from build123d import *

# Parameters (mm, degrees)
BOSS_EXTRUDE1_DEPTH = 3
FILLET1_R           = 10
FILLET2_R           = 1
FILLET3_R           = 3
SKETCH2_R           = 2.1
CUT_EXTRUDE1_DEPTH  = 42.12177039


with BuildPart() as part:
    # Sketch1 → Boss-Extrude1 (new body)
    with BuildSketch(Plane(origin=(0, 0, 0), x_dir=(1, 0, 0), z_dir=(0, 1, 0))):
        Polygon((29, -17.5), (25, -17.5), (25, -29), (-25, -29), (-25, -17.5), (-29, -17.5), (-29, 17.5), (-25, 17.5), (-25, 29), (25, 29), (25, 17.5), (29, 17.5), align=None)
    extrude(amount=BOSS_EXTRUDE1_DEPTH)

    # Fillet1
    fillet1_edges = [part.edges().sort_by_distance(p)[0] for p in [
        (25, 1.5, 29),
        (-25, 1.5, 29),
        (-25, 1.5, -29),
        (25, 1.5, -29),
    ]]
    fillet(fillet1_edges, radius=FILLET1_R)

    # Fillet2
    fillet2_edges = [part.edges().sort_by_distance(p)[0] for p in [
        (25, 1.5, 17.5),
        (-25, 1.5, 17.5),
        (-25, 1.5, -17.5),
        (25, 1.5, -17.5),
    ]]
    fillet(fillet2_edges, radius=FILLET2_R)

    # Fillet3
    fillet3_edges = [part.edges().sort_by_distance(p)[0] for p in [
        (29, 1.5, 17.5),
        (29, 1.5, -17.5),
        (-29, 1.5, 17.5),
        (-29, 1.5, -17.5),
    ]]
    fillet(fillet3_edges, radius=FILLET3_R - 0.0001)  # a hair under: the kernel refuses the full size

    # Sketch2 → Cut-Extrude1 (cut, through all)
    with BuildSketch(Plane(origin=(0, 3, 0), x_dir=(1, 0, 0), z_dir=(0, 1, 0))):
        with Locations(Location((-25.2, 0, 0), (0, 0, 270))):
            Circle(SKETCH2_R)
        with Locations(Location((25.2, 0, 0), (0, 0, 270))):
            Circle(SKETCH2_R)
    extrude(amount=-CUT_EXTRUDE1_DEPTH, mode=Mode.SUBTRACT)


solid = part.part
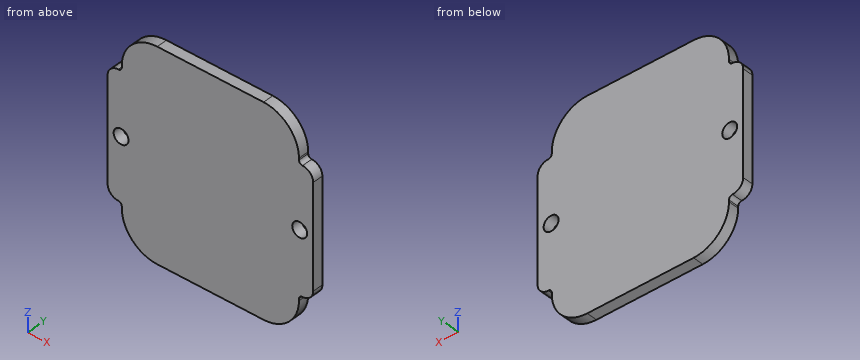
The listing builds one solid part. Answer for the finished solid, in the listing's coordinates (mm). Give positions to 0.01 mm unless a question says otherwise; leave off trailing zeros. Write each loop counter-clockwise with the first axis right and the second up, starting at its lowest first coordinate (ties: lowest second). Pieces come first, ordered by that corner, then holes.
Item 1: Section B-B, the plane y = 2 is taken. Count the separate pieces of the cut face and the enclosed holes in it, plus the area to 3 significant figures.
Item 2: A flat-ended cylindrical pin translates along its axis: P1, Ø0.6, axis at y = 2, z = 18.5, coming from the +X side. Find the tip coordinate at first contact, or state that the pin passes through.
Item 3: Find the intervals of material crossed by line 1 along X through (y, z) = (2.1, 0); line 2 along X through (y, z) = (1.4, 1); line 3 along X through (y, z) = (1.55, -15.5), in increasing order.
Item 4: Section A-A, the plane z = 0 is taken. Write down the section's boundary in (x, y), plus the area to 3 significant figures.
Item 5: Section C-C, the plane x = -19.5 is taken. Write down the section's boundary in (y, z).
Item 6: Section D-D, the plane z = 24.5 is taken. Write down the section's boundary in (x, y).
Completed:
1. separate pieces: 1
1. enclosed holes: 2
1. area: 3,060 mm2
2. P1: stops at x = 25.05
3. line 1: x = -29 to -27.3, -23.1 to 23.1, 27.3 to 29
3. line 2: x = -29 to -27.05, -23.35 to 23.35, 27.05 to 29
3. line 3: x = -28.83 to 28.83
4. outline: (-29, 0) - (-27.3, 0) - (-27.3, 3) - (-29, 3) - close; (-23.1, 0) - (23.1, 0) - (23.1, 3) - (-23.1, 3) - close; (27.3, 0) - (29, 0) - (29, 3) - (27.3, 3) - close
4. area: 149 mm2
5. outline: (0, -27.93) - (3, -27.93) - (3, 27.93) - (0, 27.93) - close
6. outline: (-23.35, 0) - (23.35, 0) - (23.35, 3) - (-23.35, 3) - close
